Verification items for this drawing (mm, ordinates from the low corner). Round coordinates to 2 decimals unless told otherwise and drop trailing zeros. Order: outer loops, then holes, each group sorted by start corner. A loop starts at its lowest first (then second) coordinate and runs counter-clockwise, first axis right, second up. Notation, with made-up numbers: (-19.75, 50) -> (-6.75, 50) arc R17 cw to (-6.75, 67) -> close; hole circle Ø5 at (33.25, 58.25). An arc over 180 degrees is marked (long way). Put each result on its own line as item: value.
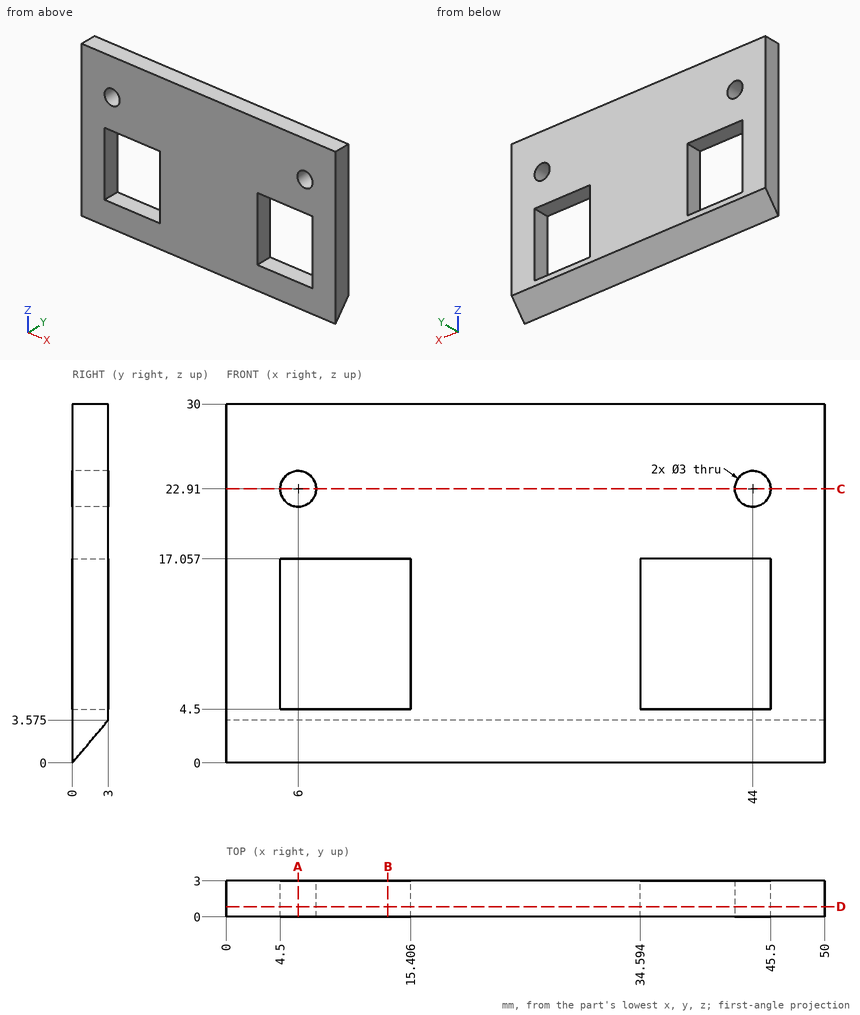
Item 1: Section check A-A on x = 6. Record the boundary of the cut face in (y, z) (1 decimal).
Check sheet entries:
outline: (0, 0) -> (3, 3.6) -> (3, 4.5) -> (0, 4.5) -> close; (0, 17.1) -> (3, 17.1) -> (3, 21.4) -> (0, 21.4) -> close; (0, 24.4) -> (3, 24.4) -> (3, 30) -> (0, 30) -> close
Item 2: Section check B-B on x = 13.5. Record the boundary of the cut face in (y, z) (1 decimal).
Check sheet entries:
outline: (0, 0) -> (3, 3.6) -> (3, 4.5) -> (0, 4.5) -> close; (0, 17.1) -> (3, 17.1) -> (3, 30) -> (0, 30) -> close
Item 3: Gauge pin test, flat ends, axial feed: pin 1 Ø2.5 at (x, z) = (44, 22.91) entering from -Y; pin 2 Ø0.9 at (x, y) = (39.5, 1.5) entering from -Z. Record the tip position at first contact, or that the pin passes through.
Check sheet entries:
pin 1: passes through
pin 2: stops at z = 1.25
Item 4: Material ranges on L1, parallel to X at y = 2.35, z = 22.91; L2, parallel to X at y = 1.4, z = 10.75; L3, parallel to Z at x = 44, y = 1.55, recorded low to high. Write a range as [from, to].
Check sheet entries:
L1: x = [0, 4.5], [7.5, 42.5], [45.5, 50]
L2: x = [0, 4.5], [15.41, 34.59], [45.5, 50]
L3: z = [1.85, 4.5], [17.06, 21.41], [24.41, 30]
Item 5: Section check C-C on z = 22.91. Record the boundary of the cut face in (x, y), then the cut area to 3 significant figures.
Check sheet entries:
outline: (0, 0) -> (4.5, 0) -> (4.5, 3) -> (0, 3) -> close; (7.5, 0) -> (42.5, 0) -> (42.5, 3) -> (7.5, 3) -> close; (45.5, 0) -> (50, 0) -> (50, 3) -> (45.5, 3) -> close
area: 132 mm^2
Item 6: Section check D-D on y = 0.85. Record the boundary of the cut face in (x, z), then the cut area to 3 significant figures.
Check sheet entries:
outline: (0, 1.01) -> (50, 1.01) -> (50, 30) -> (0, 30) -> close; hole (4.5, 4.5) -> (15.41, 4.5) -> (15.41, 17.06) -> (4.5, 17.06) -> close; hole circle Ø3 at (6, 22.91); hole (34.59, 4.5) -> (45.5, 4.5) -> (45.5, 17.06) -> (34.59, 17.06) -> close; hole circle Ø3 at (44, 22.91)
area: 1,160 mm^2
